Build history of the part. All positions in model axes, mm. Face numbers are marked on the shaded views. A direction names the side the tool comes from. Give positions to 0.01 mm unless a question says otherwise; leave off trailing zeros. Write each loop counter-clockwise with the first axis right and the second up, starting at its lowest first coordinate (ties: lowest second). Pieces come first, ordered by that corner, then holes. Notation, with made-up numbers: M -26,81.25 L 16,81.25 A17 ccw 16,109.25 Z; hole C 30.5,75 d10. An arc over 180 degrees is marked long. One line per item, written item: value. Start each with the question number.
from build123d import *

# Parameters (mm, degrees)
F0_W     = 85.2533727884
F0_H     = 80.5925950408
F1_DEPTH = 38.1
F2_W     = 45.603595674
F2_H     = 48.5711470246
F3_DEPTH = 25.4


with BuildPart() as f1:
    # F0 (on Top) → F1 (new body)
    with BuildSketch(Plane.XY):
        Rectangle(F0_W, F0_H)
    extrude(amount=F1_DEPTH)

    # F2 (on face) → F3 (cut)
    with BuildSketch(Plane.XY.offset(38.1)):
        Rectangle(F2_W, F2_H)
    extrude(amount=-F3_DEPTH, mode=Mode.SUBTRACT)

    # F4 (on face) → F6 section 0
    with BuildSketch(Plane(origin=(0, 40.2962975204, 0), x_dir=(-1, 0, 0), z_dir=(0, 1, 0))):
        with BuildLine():
            Line((18.6819845074, 38.1), (-18.6819845074, 38.1))
            ThreePointArc((-18.6819845074, 38.1), (0, 19.4180154926), (18.6819845074, 38.1))
        make_face()
    # F5 (on face) → F6 section 1
    with BuildSketch(Plane.XZ.offset(-24.2855735123)):
        with BuildLine():
            Line((6.2244155373, 38.1), (-6.2244155373, 38.1))
            ThreePointArc((-6.2244155373, 38.1), (0, 31.8755844627), (6.2244155373, 38.1))
        make_face()
    loft(mode=Mode.SUBTRACT)


solid = f1.part
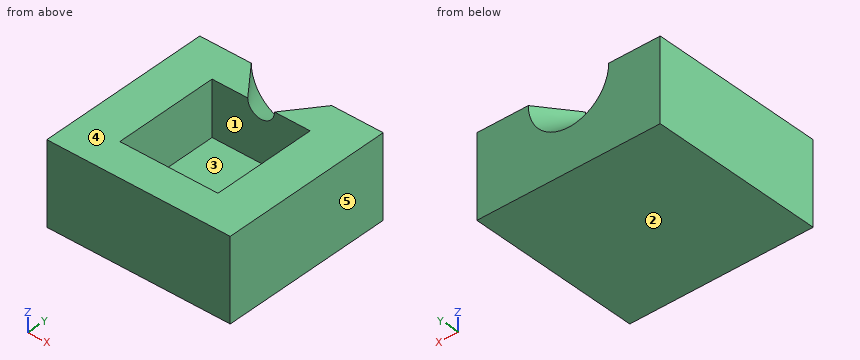
1) Mould opens along X. For the marked faces 3, 4 and 5 say: released by +X, released by -X, zero draft, split by the parting line, or undercut.
2) Band-saw the part on A-A (y = -7). List the corners of the cut face in (x, z), then the cut area to 3 significant figures.
3) Probe line 1 along X through (y, z) = (6, 19); line 2 along Y through (x, z) = (4, 17.5); line 3 along Z through (x, y) = (16.5, 21). List the from-to ranges inside material, lowest first. Write a range as from..to.
4) Band-saw the part on C-C (y = 31). List the corners of the cut face in (x, z).
5) Drop flat-ended pins along their axis: P1, Ø1.5, axis at x = 7.5, y = -2, coming from the +Z side; P2, Ø3, axis at x = 13.5, z = 31.5, coming from the +Y side. Give the stop position or say it passes through.
6) Tool access for the marked faces 1 and 2: list every direction of +Z, -Z, +X, -X, +Y, -Y with a clear straight run to the whole face (end or side of a thin tool).
7) Band-saw the part on B-B (x = 0). List the corners of the cut face in (y, z), then the cut area to 3 significant figures.
Model answer:
1. face 3: undercut
1. face 4: zero draft
1. face 5: released by +X
2. outline: M -42.63,0 L 42.63,0 L 42.63,38.1 L 22.8,38.1 L 22.8,12.7 L -22.8,12.7 L -22.8,38.1 L -42.63,38.1 Z
2. area: 2,090 mm²
3. line 1: x = -42.63..-22.8, 22.8..42.63
3. line 2: y = -40.3..-24.29, 24.29..40.3
3. line 3: z = 0..12.7
4. outline: M -42.63,0 L 42.63,0 L 42.63,38.1 L 11.45,38.1 A11.45 cw -11.45,38.1 L -42.63,38.1 Z
5. P1: stops at z = 12.7
5. P2: stops at y = 37.53
6. face 1: +Z
6. face 2: -Z, +X, -X, +Y, -Y
7. outline: M -40.3,0 L 40.3,0 L 40.3,19.42 L 24.29,31.88 L 24.29,12.7 L -24.29,12.7 L -24.29,38.1 L -40.3,38.1 Z
7. area: 1,640 mm²
